Autodesk Inventor part; units mm, degrees
ref_plane "YZ Plane" through (0, 0, 0) normal (1, 0, 0) x (0, 1, 0)
ref_plane "XZ Plane" through (0, 0, 0) normal (0, 1, 0) x (-1, 0, 0)
ref_plane "XY Plane" through (0, 0, 0) normal (0, 0, 1) x (1, 0, 0)
sketch "Sketch1" plane through (0, 0, 0) normal (0, 0, 1) x (1, 0, 0)
  line L0 (0, 0) -> (36, 0)
  line L1 (36, 0) -> (36, 30)
  line L2 (36, 30) -> (0, 30)
  line L3 (0, 30) -> (0, 0)
  circle A0 centre (10, 15) radius 2.5
  circle A1 centre (26, 15) radius 2.25
  line L4 (0, 0) -> (36, 0)
  line L5 (2, 7) -> (18, 7)
  line L6 (18, 7) -> (18, 23)
  line L7 (18, 23) -> (2, 23)
  line L8 (2, 23) -> (2, 7)
  circle A2 centre (10, 15) radius 5
  dimension "d0" = 10
  dimension "d1" = 16
  dimension "d2" = 4.5
  dimension "d3" = 5
  dimension "d4" = 15
  dimension "d5" = 15
  dimension "d6" = 10
  dimension "d7" = 15
  dimension "d15" = 10
  dimension "d16" = 8
  dimension "d17" = 8
  dimension "d18" = 8
  dimension "d19" = 8
extrude "Extrusion1" add sketch "Sketch1" against normal blind 2.5 contours L3 L2 L1 L0 | L8 L7 L6 L5 | A2
extrude "Extrusion3" add sketch "Sketch1" against normal blind 5 contours A1
extrude "Extrusion4" add sketch "Sketch1" along normal blind 5 contours L8 L7 L6 L5
chamfer "Chamfer1" distance 5 angle 45 1 edges at (18, 15, 0)
chamfer "Chamfer2" distance 5 angle 45 1 edges at (10, 7, 0)
chamfer "Chamfer4" distance 5 angle 45 1 edges at (10, 23, 0)
fillet "Fillet1" radius 5 1 edges at (36, 30, -1.25)
fillet "Fillet2" radius 5 1 edges at (0, 30, -1.25)
fillet "Fillet3" radius 5 1 edges at (36, 0, -1.25)
fillet "Fillet4" radius 5 1 edges at (0, 0, -1.25)
properties part number "keithley_2000_rear_feet"
The model under review builds one solid part; all positions refer to its coordinate system, in mm. A direction names the side the tool comes from. Give positions to 0.01 mm unless a question says otherwise; leave off trailing zeros. Write each loop counter-clockwise with the first axis right and the second up, starting at its lowest first coordinate (ties: lowest second). Pieces come first, ordered by that corner, then holes. Notation, with made-up numbers: (-5, 39) - (41, 39) arc R19 ccw to (41, 58) - close; hole circle Ø7 at (-20, 1.5). An arc over 180 degrees is marked (long way). Answer in a Markdown table with one row per item. Add a question column.
1. Draft analysis for pull direction X (two halves, no side actions). For faces 1 (the cylindrical face through (34, 29, -1)), 2 (the flat face through (12, 13, 0)), 3 (the flat face through (26, 15, -5)), state which applies: +X half, -X half, draft (parallel to the pull), parting line (faces both ways), or undercut.
2. Wall thickness on line 1 along Y through (x, z) = (10, -0.6); line 2 along Z through (x, y) = (26, 8); line 3 along Z through (x, y) = (21, 8.25): over which ranges is each line inside the solid? List them lowest first. Write a range as [from, to].
3. We need section C-C on z = -0.75. Write out the cut boundary in (x, y).
4. We need section D-D on x = 26. Write out the cut boundary in (y, z), then the cut area to 4 significant figures.
5. Tool access review of faces 4 (the cylindrical face through (2, 1, -1)), 5 (the flat face through (2, 15, 2)), 6 (the cylindrical face through (27.038, 13.004, -3.732)), 7 (the cylindrical face through (12.307, 19.436, 2.465)), 8 (the cylindrical face through (35, 2, -1)): name each direction out of +Z, -Z, +X, -X, +Y, -Y from which nothing blocks a thin tool from reaching the whole face with its end or side.
6. Insertion check: P1, Ø4, axis at y = 14.5, z = 3, coming from the -X side; P2, Ø6, axis at x = 10, y = 15, coming from the -Z side; P3, Ø1, axis at y = 15, z = 2.5, coming from the +X side. Each pin has a flat end and moves straight along its axis. Give the tip position at first contact, or say it passes through.
Ans:
| question | item | result |
|---|---|---|
| 1 | face 1 | +X half |
| 1 | face 2 | undercut |
| 1 | face 3 | draft |
| 2 | line 1 | y = [0, 12.5], [17.5, 30] |
| 2 | line 2 | z = [-2.5, 0] |
| 2 | line 3 | z = [-2.5, 2] |
| 3 | outline | (0, 5) arc R5 ccw to (5, 0) - (31, 0) arc R5 ccw to (36, 5) - (36, 25) arc R5 ccw to (31, 30) - (5, 30) arc R5 ccw to (0, 25) - close; hole circle Ø5 at (10, 15) |
| 4 | outline | (0, -2.5) - (12.75, -2.5) - (12.75, -5) - (17.25, -5) - (17.25, -2.5) - (30, -2.5) - (30, 0) - (0, 0) - close |
| 4 | area | 86.25 mm^2 |
| 5 | face 4 | +Z, -Z, -X, -Y |
| 5 | face 5 | +Z, -X, +Y, -Y |
| 5 | face 6 | -Z |
| 5 | face 7 | +Z |
| 5 | face 8 | +Z, -Z, +X, -Y |
| 6 | P1 | stops at x = 2 |
| 6 | P2 | stops at z = -2.5 |
| 6 | P3 | stops at x = 21 |
